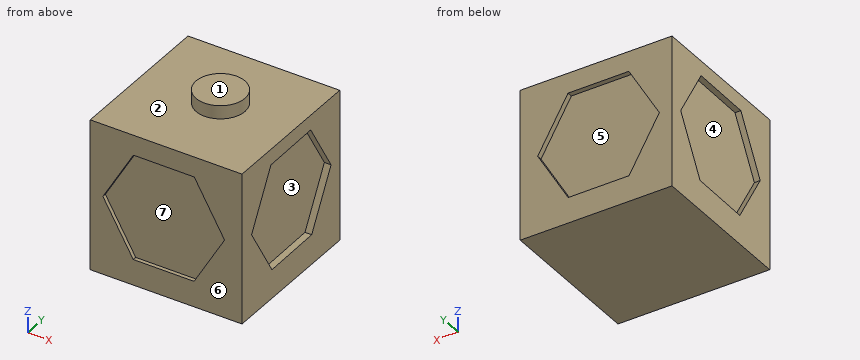
```python
from build123d import *

# Parameters (mm, degrees)
F0_W      = 100.361844
F0_H      = 100.074067
F1_DEPTH  = 100
F3_DEPTH  = 114
F4_W      = 94.14474
F4_H      = 94.934216
F5_DEPTH  = 95
F7_DEPTH  = 134
F8_W      = 92.072367
F8_H      = 92.960529
F9_DEPTH  = 94.6
F10_R     = 16.177591
F11_DEPTH = 8.8


with BuildPart() as f1:
    # F0 (on Top) → F1 (new body)
    with BuildSketch(Plane.XY):
        with Locations((-19.835529, -13.769492)):
            Rectangle(F0_W, F0_H)
    extrude(amount=F1_DEPTH)

    # F2 (on face) → F3 (cut)
    with BuildSketch(Plane.XZ.offset(63.806526)):
        Polygon((18.810559, 51.808965), (-1.24477, 86.677882), (-41.469803, 86.743916), (-61.639506, 51.941033), (-41.584177, 17.072116), (-1.359144, 17.006082), align=None)
    extrude(amount=-F3_DEPTH, mode=Mode.SUBTRACT)

    # F4 (on face) → F5 (join)
    with BuildSketch(Plane(origin=(-70.016451, 0, 0), x_dir=(0, -1, 0), z_dir=(-1, 0, 0))):
        with Locations((14.210526, 50.000002)):
            Rectangle(F4_W, F4_H)
    extrude(amount=-F5_DEPTH)

    # F6 (on face) → F7 (cut)
    with BuildSketch(Plane(origin=(-70.016451, 0, 0), x_dir=(0, -1, 0), z_dir=(-1, 0, 0))):
        Polygon((54.025555, 54.032898), (34.198133, 89.585522), (-6.505054, 90.190783), (-27.380819, 55.243419), (-7.553397, 19.690795), (33.149791, 19.085534), align=None)
    extrude(amount=-F7_DEPTH, mode=Mode.SUBTRACT)

    # F8 (on face) → F9 (join)
    with BuildSketch(Plane.XY.offset(100)):
        with Locations((-20.13158, -13.766448)):
            Rectangle(F8_W, F8_H)
    extrude(amount=-F9_DEPTH)

    # F10 (on face) → F11 (join)
    with BuildSketch(Plane.XY.offset(100)):
        with Locations((-18.50329, -10.213816)):
            Circle(F10_R)
    extrude(amount=F11_DEPTH)


solid = f1.part
```
The listing builds one solid part. Answer for the finished solid, in the listing's coordinates (mm). Face numbers are marked on the shaded views. A direction names the side the tool comes from. Give positions to 0.01 mm unless a question says otherwise; leave off trailing zeros. Write each loop counter-clockwise with the first axis right and the second up, starting at its lowest first coordinate (ties: lowest second). Pieces come first, ordered by that corner, then holes. Notation, with made-up numbers: (84.5, 37) - (97.5, 37) arc R25 cw to (97.5, 63) - close; hole circle Ø7 at (19, 73.5). An arc over 180 degrees is marked (long way). Use one line per item in the form item = value. Start each with the question number.
1) Consider line 1 along Z through (x, y) = (-55, 25.5); line 2 along Y through (x, z) = (-19.5, 40); line 3 along X through (y, z) = (-29, 33). Determine where each line is inside the solid, lowest interval first. Write a range as from..to.
2) Find section D-D on z = 82. Determine the outline of the cut face in (x, y).
3) Find section B-B on y = -48. Determine the outline of the cut face in (x, z), plus the area to 3 significant figures.
4) A tool of negligible diameter and unlimited length cuts with its end or side. For the marked faces 1, 2 and 3, from which of +Z, -Z, +X, -X, +Y, -Y can it reach the whole face along a straight path? Write none if from no direction.
5) Find section C-C on z = 64. Determine the outline of the cut face in (x, y), plus the area to 3 significant figures.
6) The mould has two halves that part along X. Classify the marked faces 4, 5, 6 and 7: pulls with the +X half, pulls with the -X half, needs draft (parallel to the pull), parting line crosses it, or undercut.
7) Find section A-A on x = -30.5. Determine the outline of the cut face in (y, z), plus the area to 3 significant figures.
8) Flat-ended cylindrical pins translate along their axes: pin 1 Ø4 at (x, z) = (-32, 56) entering from -Y; pin 2 Ø1.5 at (y, z) = (3, 32) entering from +X; pin 3 Ø6 at (y, z) = (-29, 31) entering from -X. Find the tip coordinate at first contact, or state that the pin passes through.
Geometry results:
q1.line_1 = 0..100
q1.line_2 = -61.28..32.86
q1.line_3 = -66.17..25.9
q2.outline = (-70.02, -63.81) - (-44.22, -63.81) - (-44.22, -61.28) - (1.45, -61.28) - (1.45, -63.81) - (30.35, -63.81) - (30.35, -38.43) - (25.9, -38.43) - (25.9, 11.4) - (30.35, 11.4) - (30.35, 36.27) - (1.45, 36.27) - (1.45, 32.86) - (-44.22, 32.86) - (-44.22, 36.27) - (-70.02, 36.27) - (-70.02, 11.4) - (-66.17, 11.4) - (-66.17, -38.43) - (-70.02, -38.43) - close
q3.outline = (-70.02, 0) - (30.35, 0) - (30.35, 43.95) - (25.9, 43.95) - (25.9, 64.84) - (30.35, 64.84) - (30.35, 100) - (-70.02, 100) - (-70.02, 64.84) - (-66.17, 64.84) - (-66.17, 43.95) - (-70.02, 43.95) - close
q3.area = 9,860 mm2
q4.face_1 = +Z, +X, -X, +Y, -Y
q4.face_2 = +Z
q4.face_3 = +X
q5.outline = (-70.02, -63.81) - (-54.65, -63.81) - (-54.65, -61.28) - (11.8, -61.28) - (11.8, -63.81) - (30.35, -63.81) - (30.35, -48.47) - (25.9, -48.47) - (25.9, 22.15) - (30.35, 22.15) - (30.35, 36.27) - (11.8, 36.27) - (11.8, 32.86) - (-54.65, 32.86) - (-54.65, 36.27) - (-70.02, 36.27) - (-70.02, 22.15) - (-66.17, 22.15) - (-66.17, -48.47) - (-70.02, -48.47) - close
q5.area = 9,060 mm2
q6.face_4 = pulls with the -X half
q6.face_5 = undercut
q6.face_6 = needs draft
q6.face_7 = undercut
q7.outline = (-63.81, 0) - (36.27, 0) - (36.27, 17.05) - (32.86, 17.05) - (32.86, 86.73) - (36.27, 86.73) - (36.27, 100) - (0.64, 100) - (0.64, 108.8) - (-21.07, 108.8) - (-21.07, 100) - (-63.81, 100) - (-63.81, 86.73) - (-61.28, 86.73) - (-61.28, 17.05) - (-63.81, 17.05) - close
q7.area = 9,790 mm2
q8.pin_1 = -61.28
q8.pin_2 = 25.9
q8.pin_3 = -66.17
